```python
from build123d import *

# Parameters (mm, degrees)
SKETCH1_W              = 270
SKETCH1_H              = 25
BOSS_EXTRUDE1_DEPTH    = 10
CUT_EXTRUDE1_REACH     = 273.339
SKETCH2_R              = 2.15
FILLET1_R              = 12.5
SKETCH3_R              = 2.25
CUT_EXTRUDE2_DEPTH     = 272.339271024
CUT_EXTRUDE5_REACH     = 273.339
SKETCH5_W              = 7.3
SKETCH5_H              = 4
SKETCH6_R              = 10
CUT_EXTRUDE6_DEPTH     = 5
CUT_EXTRUDE7_REACH     = 273.201
SKETCH7_R              = 1.65
CUT_EXTRUDE8_START     = -3.2
CUT_EXTRUDE8_OUTLINE_W = 6
CUT_EXTRUDE8_OUTLINE_H = 6
CUT_EXTRUDE8_DEPTH     = 6.4
SKETCH9_R              = 3
CUT_EXTRUDE9_DEPTH     = 2


# Read off the part's stored shape, not the designer's step: Cut-Extrude8
with BuildPart() as part:
    # Sketch1 → Boss-Extrude1 (new body)
    with BuildSketch(Plane(origin=(0, 0, 0), x_dir=(1, 0, 0), z_dir=(0, 1, 0))):
        with Locations((135, 12.5)):
            Rectangle(SKETCH1_W, SKETCH1_H)
    extrude(amount=BOSS_EXTRUDE1_DEPTH)

    # Sketch2 → Cut-Extrude1 (cut, up to next)
    with BuildSketch(Plane(origin=(0, 10, 0), x_dir=(1, 0, 0), z_dir=(0, 1, 0)), mode=Mode.PRIVATE) as cut_extrude1_sk1:
        with Locations(Location((12.5, 12.5, 0), (0, 0, 270))):
            Circle(SKETCH2_R)
    cut_extrude1_tool1 = extrude(cut_extrude1_sk1.sketch, amount=-CUT_EXTRUDE1_REACH, mode=Mode.PRIVATE) & part.part
    add(cut_extrude1_tool1.solids().sort_by_distance((12.5, 10, -12.5))[0], mode=Mode.SUBTRACT)

    # Fillet1
    fillet1_edges = [part.edges().sort_by_distance(p)[0] for p in [
        (0, 5, 0),
        (0, 5, -25),
    ]]
    fillet(fillet1_edges, radius=FILLET1_R - 0.0001)  # a hair under: the kernel refuses the full size

    # Sketch3 → Cut-Extrude2 (cut, through all)
    with BuildSketch(Plane(origin=(0, 0, -25), x_dir=(-1, 0, 0), z_dir=(0, 0, -1))):
        with Locations((-264.5, 5)):
            Circle(SKETCH3_R)
        with Locations((-250.5, 5)):
            Circle(SKETCH3_R)
    extrude(amount=-CUT_EXTRUDE2_DEPTH, mode=Mode.SUBTRACT)

    # Sketch5 → Cut-Extrude5 (cut, up to next)
    with BuildSketch(Plane(origin=(0, 10, 0), x_dir=(1, 0, 0), z_dir=(0, 1, 0)), mode=Mode.PRIVATE) as cut_extrude5_sk1:
        with Locations((264.5, 19)):
            Rectangle(SKETCH5_W, SKETCH5_H)
    cut_extrude5_tool1 = extrude(cut_extrude5_sk1.sketch, amount=-CUT_EXTRUDE5_REACH, mode=Mode.PRIVATE) & part.part
    # Sketch5 → Cut-Extrude5 (cut, up to next)
    with BuildSketch(Plane(origin=(0, 10, 0), x_dir=(1, 0, 0), z_dir=(0, 1, 0)), mode=Mode.PRIVATE) as cut_extrude5_sk2:
        with Locations((264.5, 6)):
            Rectangle(SKETCH5_W, SKETCH5_H)
    cut_extrude5_tool2 = extrude(cut_extrude5_sk2.sketch, amount=-CUT_EXTRUDE5_REACH, mode=Mode.PRIVATE) & part.part
    # Sketch5 → Cut-Extrude5 (cut, up to next)
    with BuildSketch(Plane(origin=(0, 10, 0), x_dir=(1, 0, 0), z_dir=(0, 1, 0)), mode=Mode.PRIVATE) as cut_extrude5_sk3:
        with Locations((250.5, 19)):
            Rectangle(SKETCH5_W, SKETCH5_H)
    cut_extrude5_tool3 = extrude(cut_extrude5_sk3.sketch, amount=-CUT_EXTRUDE5_REACH, mode=Mode.PRIVATE) & part.part
    # Sketch5 → Cut-Extrude5 (cut, up to next)
    with BuildSketch(Plane(origin=(0, 10, 0), x_dir=(1, 0, 0), z_dir=(0, 1, 0)), mode=Mode.PRIVATE) as cut_extrude5_sk4:
        with Locations((250.5, 6)):
            Rectangle(SKETCH5_W, SKETCH5_H)
    cut_extrude5_tool4 = extrude(cut_extrude5_sk4.sketch, amount=-CUT_EXTRUDE5_REACH, mode=Mode.PRIVATE) & part.part
    add(cut_extrude5_tool1.solids().sort_by_distance((264.5, 10, -19))[0], mode=Mode.SUBTRACT)
    add(cut_extrude5_tool2.solids().sort_by_distance((264.5, 10, -6))[0], mode=Mode.SUBTRACT)
    add(cut_extrude5_tool3.solids().sort_by_distance((250.5, 10, -19))[0], mode=Mode.SUBTRACT)
    add(cut_extrude5_tool4.solids().sort_by_distance((250.5, 10, -6))[0], mode=Mode.SUBTRACT)

    # Sketch6 → Cut-Extrude6 (cut)
    with BuildSketch(Plane.XZ):
        with Locations(Location((12.5, -12.5, 0), (0, 0, 270))):
            Circle(SKETCH6_R)
    extrude(amount=-CUT_EXTRUDE6_DEPTH, mode=Mode.SUBTRACT)

    # Sketch7 → Cut-Extrude7 (cut, up to next)
    with BuildSketch(Plane.XZ.offset(-5), mode=Mode.PRIVATE) as cut_extrude7_sk1:
        with Locations(Location((12.5, -6, 0), (0, 0, 270))):
            Circle(SKETCH7_R)
    cut_extrude7_tool1 = extrude(cut_extrude7_sk1.sketch, amount=-CUT_EXTRUDE7_REACH, mode=Mode.PRIVATE) & part.part
    # Sketch7 → Cut-Extrude7 (cut, up to next)
    with BuildSketch(Plane.XZ.offset(-5), mode=Mode.PRIVATE) as cut_extrude7_sk2:
        with Locations(Location((19, -12.5, 0), (0, 0, 270))):
            Circle(SKETCH7_R)
    cut_extrude7_tool2 = extrude(cut_extrude7_sk2.sketch, amount=-CUT_EXTRUDE7_REACH, mode=Mode.PRIVATE) & part.part
    # Sketch7 → Cut-Extrude7 (cut, up to next)
    with BuildSketch(Plane.XZ.offset(-5), mode=Mode.PRIVATE) as cut_extrude7_sk3:
        with Locations(Location((12.5, -19, 0), (0, 0, 270))):
            Circle(SKETCH7_R)
    cut_extrude7_tool3 = extrude(cut_extrude7_sk3.sketch, amount=-CUT_EXTRUDE7_REACH, mode=Mode.PRIVATE) & part.part
    # Sketch7 → Cut-Extrude7 (cut, up to next)
    with BuildSketch(Plane.XZ.offset(-5), mode=Mode.PRIVATE) as cut_extrude7_sk4:
        with Locations(Location((6, -12.5, 0), (0, 0, 270))):
            Circle(SKETCH7_R)
    cut_extrude7_tool4 = extrude(cut_extrude7_sk4.sketch, amount=-CUT_EXTRUDE7_REACH, mode=Mode.PRIVATE) & part.part
    add(cut_extrude7_tool1.solids().sort_by_distance((12.5, 5, -6))[0], mode=Mode.SUBTRACT)
    add(cut_extrude7_tool2.solids().sort_by_distance((19, 5, -12.5))[0], mode=Mode.SUBTRACT)
    add(cut_extrude7_tool3.solids().sort_by_distance((12.5, 5, -19))[0], mode=Mode.SUBTRACT)
    add(cut_extrude7_tool4.solids().sort_by_distance((6, 5, -12.5))[0], mode=Mode.SUBTRACT)

    # Cut-Extrude8 outline → Cut-Extrude8 (cut)
    with BuildSketch(Plane(origin=(0, 0, 0), x_dir=(0.707106781186548, 0, -0.707106781186547), z_dir=(0.707106781186547, 0, 0.707106781186548)).offset(CUT_EXTRUDE8_START)):
        with Locations((7, 2)):
            Rectangle(CUT_EXTRUDE8_OUTLINE_W, CUT_EXTRUDE8_OUTLINE_H)
    extrude(amount=CUT_EXTRUDE8_DEPTH, mode=Mode.SUBTRACT)

    # Sketch9 → Cut-Extrude9 (cut)
    with BuildSketch(Plane(origin=(0, 10, 0), x_dir=(1, 0, 0), z_dir=(0, 1, 0))):
        with Locations(Location((12.5, 19, 0), (0, 0, 270))):
            Circle(SKETCH9_R)
        with Locations(Location((19, 12.5, 0), (0, 0, 270))):
            Circle(SKETCH9_R)
        with Locations(Location((12.5, 6, 0), (0, 0, 270))):
            Circle(SKETCH9_R)
        with Locations(Location((6, 12.5, 0), (0, 0, 270))):
            Circle(SKETCH9_R)
    extrude(amount=-CUT_EXTRUDE9_DEPTH, mode=Mode.SUBTRACT)


solid = part.part
```
CAD build for the part. Positions are in the model's coordinates, mm. A direction names the side the tool comes from. Coordinates: 2 decimals unless noted, no trailing zeros. Write each loop counter-clockwise with the first axis right and the second up, starting at its lowest first coordinate (ties: lowest second). Pieces come first, ordered by that corner, then holes. Notation, with made-up numbers: (31, 88.25) -> (40, 88.25) arc R33 cw to (40, 116.25) -> close; hole circle Ø10 at (-10.5, 57.25). An arc over 180 degrees is marked (long way). Use CSV: the item, a comma, the result in double quotes. Start each with the question number.
Item 1: Drop flat-ended pins along their axis: P1, Ø4.5, axis at y = 5.5, z = -20, coming from the -X side; P2, Ø2, axis at y = 6.5, z = -19.5, coming from the -X side; P3, Ø5.5, axis at x = 12.5, z = -6, coming from the +Y side; P4, Ø3, axis at x = 6, z = -12.5, coming from the +Y side. Give the stop position or say it passes through.
Item 2: Band-saw the part on A-A, the plane x = 264.5. Write the cut outline in (y, z), plus the area to 3 significant figures.
Item 3: Tool access for faces 1 (the flat face through (139, 5, -25)), 2 (the cylindrical face through (19.29, 2.46, -19.84)), 3 (the flat face through (251.3, 7.3, -8)), 4 (the cylindrical face through (4.2, 9, -14.9)): list every direction of +Z, -Z, +X, -X, +Y, -Y with a clear straight run to the whole face (end or side of a thin tool).
Item 4: Wall check: probe 1 along Y at (x, z) = (250.5, -22.35); probe 2 along Z at (x, y) = (12.5, 3.75); probe 3 along X at (y, z) = (8.8, -12.5). Give the ranges that are in metal, low to high.
Item 5: Two-plate mould, pull along X, no slides. Class faces 5 (the cylindrical face through (13.4, 9.01, -3.14)), 6 (the cylindrical face through (17.2, 9, -14.9)), 7 (the cylindrical face through (3.564, 6.181, -3.759)), 8 (the flat face through (133, 0, -13)): +X half, -X half, draft (parallel to the pull), parting line (faces both ways), or undercut.
Response values:
1,P1,"stops at x = 1.16"
1,P2,"stops at x = 1.53"
1,P3,"stops at y = 8"
1,P4,"passes through"
2,outline,"(0, -25) -> (2.75, -25) -> (2.75, -21) -> (0, -21) -> close; (0, -17) -> (2.75, -17) -> (2.75, -8) -> (0, -8) -> close; (0, -4) -> (2.75, -4) -> (2.75, 0) -> (0, 0) -> close; (7.25, -25) -> (10, -25) -> (10, -21) -> (7.25, -21) -> close; (7.25, -17) -> (10, -17) -> (10, -8) -> (7.25, -8) -> close; (7.25, -4) -> (10, -4) -> (10, 0) -> (7.25, 0) -> close"
2,area,"93.5 mm2"
3,face 1,"-Z, +X, -X, +Y, -Y"
3,face 2,"-Y"
3,face 3,"+Y, -Y"
3,face 4,"+Y"
4,probe 1,"y = 0 to 2.75, 7.25 to 10"
4,probe 2,"z = -25 to -22.5, -2.5 to 0"
4,probe 3,"x = 0 to 3, 9 to 10.35, 14.65 to 16, 22 to 270"
5,face 5,"undercut"
5,face 6,"undercut"
5,face 7,"-X half"
5,face 8,"draft"
